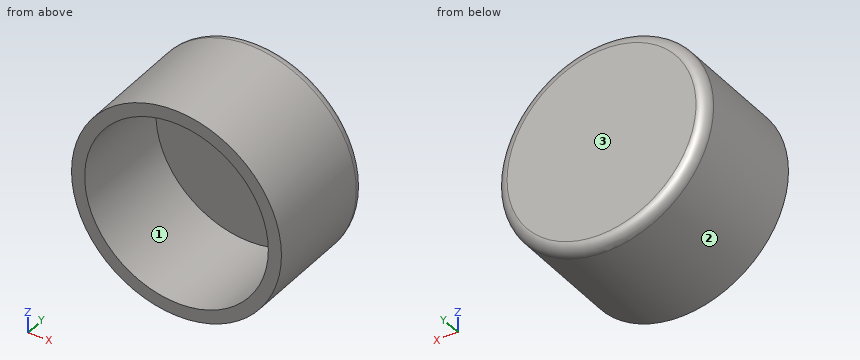
from build123d import *

# Parameters (mm, degrees)
SKETCH2_R           = 50.8
SKETCH2_R_2         = 44.45
BOSS_EXTRUDE2_DEPTH = 50.8
SKETCH6_R           = 50.8
BOSS_EXTRUDE3_DEPTH = 7.62
FILLET1_R           = 5.08


with BuildPart() as part:
    # Sketch2 → Boss-Extrude2 (new body)
    with BuildSketch(Plane(origin=(0, 0, 0), x_dir=(1, 0, 0), z_dir=(0, 1, 0))):
        Circle(SKETCH2_R)
        Circle(SKETCH2_R_2, mode=Mode.SUBTRACT)
    extrude(amount=BOSS_EXTRUDE2_DEPTH)

    # Sketch6 → Boss-Extrude3 (add)
    with BuildSketch(Plane(origin=(0, 50.8, 0), x_dir=(1, 0, 0), z_dir=(0, 1, 0))):
        Circle(SKETCH6_R)
    extrude(amount=BOSS_EXTRUDE3_DEPTH)

    # Fillet1
    fillet1_edges = [part.edges().sort_by_distance(p)[0] for p in [
        (-50.8, 58.42, 0),
    ]]
    fillet(fillet1_edges, radius=FILLET1_R)


solid = part.part
Model file for the job. Use its own axes, mm. Face numbers are marked on the shaded views. Give positions to 0.01 mm unless a question says otherwise; leave off trailing zeros. Order: outer loops, then holes, each group sorted by start corner. A loop starts at its lowest first (then second) coordinate and runs counter-clockwise, first axis right, second up. Notation, with made-up numbers: M 28.5,38 L 69.5,38 A24 ccw 69.5,48 Z; hole C -29.75,39.5 d5. An arc over 180 degrees is marked long. Put each result on its own line as item: value. Start each with the question number.
(1) Band-saw the part on B-B on x = 0. Give the cut face in (y, z), then the cut area to 3 significant figures.
(2) Band-saw the part on A-A on z = 0. Give the cut face in (x, y).
(3) Pin check, flat tips, straight feed: pin 1 Ø1 at (y, z) = (49, -14.5) entering from +X; pin 2 Ø8 at (x, y) = (-6.5, 15.5) entering from +Z; pin 3 Ø8 at (x, z) = (4, -35) entering from -Y. Stop position of each tip, or through.
(4) Drill centre lines: L1, parallel to Z at x = 0, y = 12; L2, parallel to Y at x = -3.5, z = -4; L3, parallel to X at y = 18.5, z = -36.5. Where is each one in solid material? Low to high. Write a range as [from, to].
(5) Pull direction Z, two halves, no side cores. Call the marked faces 1, 2 and 3: released by +Z, released by -Z, zero draft, split by the parting line, or undercut.
(6) Band-saw the part on C-C on y = 13.5. Give the cut face in (x, z), then the cut area to 3 significant figures.
Results below:
1. outline: M 0,-50.8 L 53.34,-50.8 A5.08 ccw 58.42,-45.72 L 58.42,45.72 A5.08 ccw 53.34,50.8 L 0,50.8 L 0,44.45 L 50.8,44.45 L 50.8,-44.45 L 0,-44.45 Z
1. area: 1,410 mm2
2. outline: M -50.8,0 L -44.45,0 L -44.45,50.8 L 44.45,50.8 L 44.45,0 L 50.8,0 L 50.8,53.34 A5.08 ccw 45.72,58.42 L -45.72,58.42 A5.08 ccw -50.8,53.34 Z
3. pin 1: stops at x = 48.83
3. pin 2: stops at z = 50.74
3. pin 3: stops at y = 50.8
4. L1: z = [-50.8, -44.45], [44.45, 50.8]
4. L2: y = [50.8, 58.42]
4. L3: x = [-35.33, -25.37], [25.37, 35.33]
5. face 1: undercut
5. face 2: split by the parting line
5. face 3: zero draft
6. outline: C 0,0 d101.6; hole C 0,0 d88.9
6. area: 1,900 mm2
